Autodesk Inventor part; units mm, degrees
ref_plane "YZ Plane" through (0, 0, 0) normal (1, 0, 0) x (0, 1, 0)
ref_plane "XZ Plane" through (0, 0, 0) normal (0, 1, 0) x (-1, 0, 0)
ref_plane "XY Plane" through (0, 0, 0) normal (0, 0, 1) x (1, 0, 0)
sketch "Sketch1" plane through (0, 0, 0) normal (0, 0, 1) x (1, 0, 0)
  line L0 (0, 0) -> (-179.6388, 0)
  line L1 (-179.6388, 0) -> (-179.6388, -1500)
  line L2 (-179.6388, -1500) -> (0, -1500)
  line L3 (0, -1500) -> (0, 0)
  line L4 (-179.6388, -1400) -> (-81, -1400)
  line L5 (-81, -1400) -> (-81, -1394)
  line L6 (-81, -1394) -> (-179.6388, -1394)
  line L7 (-179.6388, -1394) -> (-179.6388, -1400)
  line L8 (-179.6388, -900) -> (-81, -900)
  line L9 (-81, -900) -> (-81, -894)
  line L10 (-81, -894) -> (-179.6388, -894)
  line L11 (-179.6388, -894) -> (-179.6388, -900)
  line L12 (-179.6388, -400) -> (-81, -400)
  line L13 (-81, -400) -> (-81, -394)
  line L14 (-81, -394) -> (-179.6388, -394)
  line L15 (-179.6388, -394) -> (-179.6388, -400)
  point P0 (-179.6388, -394)
  point P1 (-179.6388, -400)
  point P2 (-179.6388, -1394)
  dimension "d0" = 1500
  dimension "d1" = 179.6388
  dimension "d2" = 6
  dimension "d4" = 100
  dimension "d7" = 500
  dimension "d23" = 81
extrude "Plate1" add sketch "Sketch1" along normal blind 4 contours L3 L2 L1 L4 L5 L6 L8 L9 L10 L12 L13 L14 L0
sketch "Sketch2" plane through (4, 0, 0) normal (-1, 0, 0) x (0, -1, 0)
  line L0 (1500, 0) -> (0, 0)
  line L1 (0, 0) -> (0, 35)
  line L2 (0, 35) -> (1500, 35)
  line L3 (1500, 35) -> (1500, 0)
edge flange "Flange1" height 35 angle 90 thickness 4 bend radius 4 thickness toward (-1, 0, 0) relief tear relief width 4 relief depth 2 edges at (0, -750, 4) wall of the first edge with corners at (4, -1500, 0) (4, 0, 0) (4, 0, 35) (4, -1500, 35)
bend "Bend1"
corner "Corner1"
equation "\"d1\" = Stringer2_deep"
equation "\"d12\" = Thickness"
equation "\"d13\" = BendReliefWidth"
equation "\"d14\" = BendReliefDepth"
equation "\"d15\" = MinimumRemnant"
equation "\"d16\" = TransitionRadius"
equation "\"d19\" = BendRadius"
equation "\"d20\" = CornerReliefSize"
equation "\"d21\" = GapSize"
equation "\"d22\" = JacobiRadiusSize"
equation "\"BendRadius\" = Thickness"
equation "\"BendReliefWidth\" = Thickness"
equation "\"BendReliefDepth\" = 0.5 * Thickness"
equation "\"CornerReliefSize\" = 4 * Thickness"
equation "\"MinimumRemnant\" = 2 * Thickness"
equation "\"TransitionRadius\" = BendRadius"
equation "\"JacobiRadiusSize\" = BendRadius"
equation "\"GapSize\" = Thickness"
properties part number "stringer 1.2" material "Steel"
Geometry: final body of the model. Coordinates: model frame, mm. A direction names the side the tool comes from. Round coordinates to 2 decimals unless told otherwise and drop trailing zeros. Loops run counter-clockwise (first coordinate to the right, second up) from the corner with the lowest first, then second, coordinate; pieces in that order, holes last. Notation, with made-up numbers: M -9.75,-36.5 L 0.25,-36.5 A11 ccw 0.25,-16.5 Z; hole C 83,-9.5 d2. An arc over 180 degrees is marked long. One line per question, with ' | ' between items.
(1) Cut plane B-B on y = -433. Return the cut outline in (x, z).
Check result:
outline: M -179.64,0 L -4,0 A8 ccw 4,8 L 4,35 L 0,35 L 0,8 A4 cw -4,4 L -179.64,4 Z
(2) Cut plane A-A on x = -132. Return the cut outline in (y, z).
Check result:
outline: M -1500,0 L -1400,0 L -1400,4 L -1500,4 Z; M -1394,0 L -900,0 L -900,4 L -1394,4 Z; M -894,0 L -400,0 L -400,4 L -894,4 Z; M -394,0 L 0,0 L 0,4 L -394,4 Z
(3) Material intervals for line 1 along Y through (x, z) = (-130, 2.5); line 2 along Z through (x, y) = (-136, -755.5), sorted ascending. Write a range as from..to.
Check result:
line 1: y = -1500..-1400, -1394..-900, -894..-400, -394..0 | line 2: z = 0..4
(4) Cut plane D-D on z = 19. Return the cut outline in (x, y).
Check result:
outline: M 0,-1500 L 4,-1500 L 4,0 L 0,0 Z
(5) Access query for faces 1 (the flat face through (-93, -740, 4)), 2 (the flat face through (-67, -1500, 3)). Directions: +Z, -Z, +X, -X, +Y, -Y. A direction counts if a zero-diameter tool reaches every point of the face in a straight line with its end or side. Return the directions, or none.
Check result:
face 1: +Z, -X, +Y, -Y | face 2: +Z, -Z, +X, -X, -Y
(6) Contact query for flat-ended pins moving along their axis: P1, Ø1.2, axis at y = -896.5, z = 2, coming from the -X side; P2, Ø13.5, axis at y = -1020, z = 18.5, coming from the -X side; P3, Ø4, axis at x = -24, y = -1125, coming from the +Z side. Output: stop coordinate, or through.
Check result:
P1: stops at x = -81 | P2: stops at x = 0 | P3: stops at z = 4
(7) Cut plane C-C on x = -52. Return the cut outline in (y, z), plus the area to 3 significant figures.
Check result:
outline: M -1500,0 L 0,0 L 0,4 L -1500,4 Z | area: 6,000 mm2
